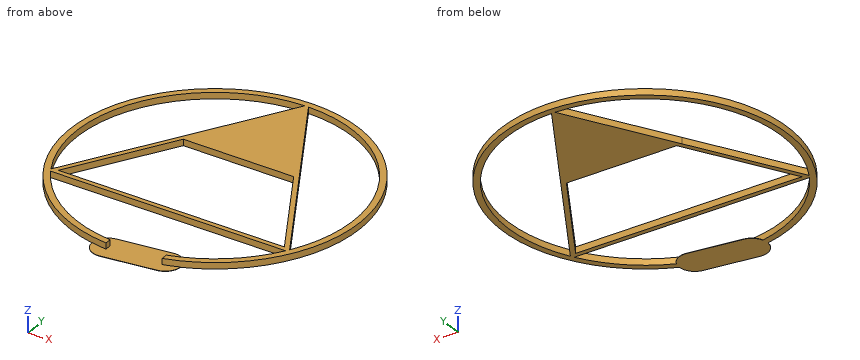
from build123d import *

# Parameters (mm, degrees)
F0_R     = 46
F1_DEPTH = 1
F2_W     = 17
F2_H     = 23.0149852611
F3_DEPTH = 12.5
F5_START = -0.9
F5_DEPTH = 0.1


with BuildPart() as f1:
    # F0 (on Top) → F1 (new body, symmetric)
    with BuildSketch(Plane.XY):
        Circle(F0_R)
        with BuildLine():
            ThreePointArc((0, 45), (31.8198051534, 31.8198051534), (45, 0))
            ThreePointArc((45, 0), (43.466662183, -11.6468570296), (38.9711431703, -22.5))
            ThreePointArc((38.9711431703, -22.5), (0, -45), (-38.9711431703, -22.5))
            ThreePointArc((-38.9711431703, -22.5), (-38.9711431703, 22.5), (0, 45))
        make_face(mode=Mode.SUBTRACT)
        with BuildLine():
            Line((-0.5795540246, 43.9961829837), (0, 45))
            ThreePointArc((0, 45), (-38.9711431703, 22.5), (-38.9711431703, -22.5))
            Line((-38.9711431703, -22.5), (-38.3915891457, -21.4961829837))
            ThreePointArc((-38.3915891457, -21.4961829837), (-38.1051177665, 22), (-0.5795540246, 43.9961829837))
        make_face()
        with BuildLine():
            ThreePointArc((37.8120351211, -22.5), (38.1051177665, -22), (38.3915891457, -21.4961829837))
            Line((38.3915891457, -21.4961829837), (19.4855715851, 11.25))
            Line((19.4855715851, 11.25), (17.7535207776, 11.25))
            Line((17.7535207776, 11.25), (36.3730669589, -21))
            Line((36.3730669589, -21), (-36.3730669589, -21))
            Line((-36.3730669589, -21), (-17.7535207776, 11.25))
            Line((-17.7535207776, 11.25), (-19.4855715851, 11.25))
            Line((-19.4855715851, 11.25), (-38.3915891457, -21.4961829837))
            ThreePointArc((-38.3915891457, -21.4961829837), (-38.1051177665, -22), (-37.8120351211, -22.5))
            Line((-37.8120351211, -22.5), (37.8120351211, -22.5))
        make_face()
        with BuildLine():
            Line((19.4855715851, 11.25), (0.5795540246, 43.9961829837))
            ThreePointArc((0.5795540246, 43.9961829837), (0, 44), (-0.5795540246, 43.9961829837))
            Line((-0.5795540246, 43.9961829837), (-19.4855715851, 11.25))
            Line((-19.4855715851, 11.25), (-17.7535207776, 11.25))
            Line((-17.7535207776, 11.25), (0, 42))
            Line((0, 42), (17.7535207776, 11.25))
            Line((17.7535207776, 11.25), (19.4855715851, 11.25))
        make_face()
        with BuildLine():
            ThreePointArc((38.9711431703, -22.5), (43.466662183, -11.6468570296), (45, 0))
            ThreePointArc((45, 0), (31.8198051534, 31.8198051534), (0, 45))
            Line((0, 45), (0.5795540246, 43.9961829837))
            ThreePointArc((0.5795540246, 43.9961829837), (31.3169313398, 30.9071158709), (44, 0))
            ThreePointArc((44, 0), (42.5748160443, -11.107881832), (38.3915891457, -21.4961829837))
            Line((38.3915891457, -21.4961829837), (38.9711431703, -22.5))
        make_face()
        with BuildLine():
            ThreePointArc((-38.9711431703, -22.5), (0, -45), (38.9711431703, -22.5))
            Line((38.9711431703, -22.5), (37.8120351211, -22.5))
            ThreePointArc((37.8120351211, -22.5), (0, -44), (-37.8120351211, -22.5))
            Line((-37.8120351211, -22.5), (-38.9711431703, -22.5))
        make_face()
        with BuildLine():
            Line((37.8120351211, -22.5), (38.9711431703, -22.5))
            Line((38.9711431703, -22.5), (38.3915891457, -21.4961829837))
            ThreePointArc((38.3915891457, -21.4961829837), (38.1051177665, -22), (37.8120351211, -22.5))
        make_face()
        with BuildLine():
            Line((0.5795540246, 43.9961829837), (0, 45))
            Line((0, 45), (-0.5795540246, 43.9961829837))
            ThreePointArc((-0.5795540246, 43.9961829837), (0, 44), (0.5795540246, 43.9961829837))
        make_face()
        with BuildLine():
            Line((-38.3915891457, -21.4961829837), (-38.9711431703, -22.5))
            Line((-38.9711431703, -22.5), (-37.8120351211, -22.5))
            ThreePointArc((-37.8120351211, -22.5), (-38.1051177665, -22), (-38.3915891457, -21.4961829837))
        make_face()
        Polygon((-17.7535207776, 11.25), (17.7535207776, 11.25), (0, 42), align=None)
    extrude(amount=F1_DEPTH, both=True)

    # F2 (on Top) → F3 (cut, symmetric)
    with BuildSketch(Plane.XY):
        with Locations((4.1, -46.7491300095)):
            Rectangle(F2_W, F2_H)
    extrude(amount=F3_DEPTH, both=True, mode=Mode.SUBTRACT)

    # F4 (on Top) → F5 (join)
    with BuildSketch(Plane.XY.offset(F5_START)):
        with BuildLine():
            ThreePointArc((-3.73206699, -49.7394501678), (-0.6357162003, -48.0751864298), (0.6, -44.7842644504))
            ThreePointArc((0.6, -44.7842644504), (-1.1090780205, -41.0199806506), (-5.06793301, -39.8290787329))
            ThreePointArc((-5.06793301, -39.8290787329), (-9.3551857174, -45.4521974603), (-3.73206699, -49.7394501678))
        make_face()
        with BuildLine():
            ThreePointArc((-5.06793301, -39.8290787329), (-1.1090780205, -41.0199806506), (0.6, -44.7842644504))
            ThreePointArc((0.6, -44.7842644504), (-0.6357162003, -48.0751864298), (-3.73206699, -49.7394501678))
            Line((-3.73206699, -49.7394501678), (13.1197539442, -47.4679132119))
            ThreePointArc((13.1197539442, -47.4679132119), (7.4966352168, -43.1806605044), (11.7838879242, -37.557541777))
            Line((11.7838879242, -37.557541777), (-5.06793301, -39.8290787329))
        make_face()
        with BuildLine():
            ThreePointArc((17.4518209342, -42.5127274945), (15.7427429137, -38.7484436947), (11.7838879242, -37.557541777))
            ThreePointArc((11.7838879242, -37.557541777), (7.4966352168, -43.1806605044), (13.1197539442, -47.4679132119))
            ThreePointArc((13.1197539442, -47.4679132119), (16.216104734, -45.8036494739), (17.4518209342, -42.5127274945))
        make_face()
    extrude(amount=-F5_DEPTH)


solid = f1.part
CAD build for the part. Positions are in the model's coordinates, mm. Coordinates: 2 decimals unless noted, no trailing zeros. Loops run counter-clockwise (first coordinate to the right, second up) from the corner with the lowest first, then second, coordinate; pieces in that order, holes last. Notation, with made-up numbers: (-30.75, -21) - (3.25, -21) arc R16 cw to (3.25, 7) - close; hole circle Ø10 at (75.25, -24.5). An arc over 180 degrees is marked (long way). Use one line per item in the form item = value. Start each with the question number.
1) Band-saw the part on D-D (y = 1.5). Give the cut face in (x, z).
2) Band-saw the part on C-C (z = -0.45). Give the cut face in (x, y), and give its area (3 significant figures).
3) Band-saw the part on B-B (y = -34.5). Give the cut face in (x, z).
4) Flat gauge pins, fed straight in: pin 1 (0.6 mm diameter, centred on y = -45, z = 0, fed in from +X); pin 2 (3.5 mm diameter, centred on x = -1.5, y = -43.5, fed in from +Z); pin 3 (0.6 mm diameter, centred on x = -17, z = 0, fed in from -Y). Where does each tip first touch, or does it go through?
5) Band-saw the part on A-A (x = -25.5). Give the cut face in (y, z).
6) Drill centre lines: L1, parallel to Y at x = -8.5, z = -0.7; L2, parallel to Y at x = 2, z = -0.35; L3, parallel to X at y = -5.5, z = 0.85. Where is each one in solid material? Low to high. Write a range as from..to.
Check values:
q1.outline = (-45.98, -1) - (-43.97, -1) - (-43.97, 1) - (-45.98, 1) - close; (-25.11, -1) - (-23.38, -1) - (-23.38, 1) - (-25.11, 1) - close; (23.38, -1) - (25.11, -1) - (25.11, 1) - (23.38, 1) - close; (43.97, -1) - (45.98, -1) - (45.98, 1) - (43.97, 1) - close
q2.outline = (-37.81, -22.5) - (37.81, -22.5) arc R44 cw to (12.6, -42.16) - (12.6, -44.24) arc R46 ccw (long way) to (-4.4, -45.79) - (-4.4, -43.78) arc R44 cw to start; hole (-38.39, -21.5) - (-0.58, 44) arc R44 ccw to start; hole (-36.37, -21) - (36.37, -21) - (17.75, 11.25) - (-17.75, 11.25) - close; hole (0.58, 44) - (38.39, -21.5) arc R44 ccw to start
q2.area = 1,410 mm2
q3.outline = (-30.43, -1) - (-27.31, -1) - (-27.31, 1) - (-30.43, 1) - close; (27.31, -1) - (30.43, -1) - (30.43, 1) - (27.31, 1) - close
q4.pin_1 = -4.4
q4.pin_2 = -0.9
q4.pin_3 = -42.86
q5.outline = (-38.29, -1) - (-35.86, -1) - (-35.86, 1) - (-38.29, 1) - close; (-22.5, -1) - (-21, -1) - (-21, 1) - (-22.5, 1) - close; (-2.17, -1) - (0.83, -1) - (0.83, 1) - (-2.17, 1) - close; (35.86, -1) - (38.29, -1) - (38.29, 1) - (35.86, 1) - close
q6.L1 = -45.21..-43.17, -22.5..-21, 11.25..30.28, 43.17..45.21
q6.L2 = -22.5..-21, 11.25..41.54, 43.95..45.96
q6.L3 = -45.67..-43.65, -29.16..-27.42, 27.42..29.16, 43.65..45.67
